Autodesk Inventor part; units mm, degrees
ref_plane "YZ Plane" through (0, 0, 0) normal (1, 0, 0) x (0, 1, 0)
ref_plane "XZ Plane" through (0, 0, 0) normal (0, 1, 0) x (-1, 0, 0)
ref_plane "XY Plane" through (0, 0, 0) normal (0, 0, 1) x (1, 0, 0)
sketch "Sketch1" plane through (0, 0, 0) normal (0, 0, 1) x (1, 0, 0)
  line L0 (49.9773, 11) -> (55.5082, 11)
  line L1 (-0.0227, 11) -> (-0.0227, 17)
  line L2 (-0.0227, 11) -> (-0.0227, 17)
  line L3 (-0.0227, 11) -> (-0.0227, 17)
  line L4 (-0.0227, 17) -> (55.5082, 17)
  line L5 (55.5082, 17) -> (55.5082, -83)
  line L6 (55.5082, -83) -> (-0.0227, -83)
  line L7 (-0.0227, -83) -> (-0.0227, 17)
  line L8 (55.5082, 17) -> (55.5082, 11)
  line L9 (55.5082, 17) -> (55.5082, 11)
  dimension "d16" = 100
extrude "Extrusion1" add sketch "Sketch1" along normal blind 6
sketch "Sketch2" plane through (0, 0, 6) normal (0, 0, 1) x (1, 0, 0)
  line L0 (49.9773, 11) -> (55.5082, 11)
  line L1 (49.9773, 17) -> (49.9773, 11)
  line L2 (29.9773, 17) -> (29.9773, 11)
  line L3 (29.9773, 11) -> (39.9773, 11)
  line L4 (39.9773, 11) -> (39.9773, 17)
  line L5 (49.9773, 11) -> (49.8773, 11)
  line L6 (49.8773, 11) -> (49.8773, 17)
  line L7 (49.8773, 17) -> (49.9773, 17)
  line L8 (49.9773, 17) -> (49.9773, 11)
  line L9 (39.9773, 11) -> (40.0773, 11)
  line L10 (40.0773, 11) -> (40.0773, 17)
  line L11 (40.0773, 17) -> (39.9773, 17)
  line L12 (39.9773, 17) -> (39.9773, 11)
  line L13 (29.9773, 11) -> (29.8773, 11)
  line L14 (29.8773, 11) -> (29.8773, 17)
  line L15 (29.8773, 17) -> (29.9773, 17)
  line L16 (29.9773, 17) -> (29.9773, 11)
  line L17 (9.9773, 17) -> (9.9773, 11)
  line L18 (19.9773, 11) -> (19.9773, 17)
  line L19 (9.9773, 11) -> (19.9773, 11)
  line L20 (19.9773, 11) -> (20.0773, 11)
  line L21 (20.0773, 11) -> (20.0773, 17)
  line L22 (20.0773, 17) -> (19.9773, 17)
  line L23 (19.9773, 17) -> (19.9773, 11)
  line L24 (9.9773, 11) -> (9.8773, 11)
  line L25 (9.8773, 11) -> (9.8773, 17)
  line L26 (9.8773, 17) -> (9.9773, 17)
  line L27 (9.9773, 17) -> (9.9773, 11)
  line L28 (55.5082, -83) -> (55.5082, 17)
  line L29 (39.9773, 11) -> (29.9773, 11)
  line L30 (19.9773, 11) -> (9.9773, 11)
  line L31 (49.9773, 11) -> (55.5082, 11)
  line L32 (-0.0227, 17) -> (-0.0227, -83)
  line L33 (55.5082, 17) -> (-0.0227, 17)
  point P0 (49.9, 0.06)
  point P1 (30.1, 0)
  point P2 (39.9, 0)
  point P3 (39.9, 0.03)
  point P4 (30.1, 2.97)
  point P5 (40, 0)
  point P6 (40, 0)
  point P7 (9.9773, 17)
  point P8 (19.9773, 17)
  point P9 (9.9773, 17)
  point P10 (39.9773, 17)
  point P11 (29.9773, 17)
  point P12 (49.9773, 17)
  dimension "d3" = 0.1
  dimension "d4" = 6
  dimension "d5" = 0.1
  dimension "d6" = 6
  dimension "d7" = 0.1
  dimension "d8" = 6
  dimension "d17" = 0.1
  dimension "d18" = 6
  dimension "d19" = 0.1
  dimension "d20" = 6
extrude "Extrusion2" cut sketch "Sketch2" against normal through all contours L5 L6 L7 L1 | L21 L20 L18 L22 | L4 L3 L2 L33 | L2 L13 L14 L15 | L18 L19 L17 L33 | L17 L24 L25 L26
ref_plane "Work Plane1" through (-0.0227, -33, 0) normal (0, -1, 0) x (1, 0, 0)
mirror "Mirror1" about plane through (-0.0227, -33, 0) normal (0, -1, 0) of "Extrusion2"
sketch "Sketch3" plane through (0, 0, 6) normal (0, 0, 1) x (1, 0, 0)
  line L0 (37.75, -5.4) -> (32.25, -5.4)
  line L1 (32.25, -5.4) -> (32.25, -3)
  line L2 (32.25, -3) -> (37.75, -3)
  line L3 (37.75, -3) -> (37.75, -5.4)
  line L4 (40.1, 7.6673) -> (40.1, 6)
  line L5 (40.1, 0) -> (29.9, 0)
  point P0 (0, 0)
  dimension "d21" = 5.5
  dimension "d22" = 2.4
  dimension "d23" = 2.35
  dimension "d24" = 3
extrude "Extrusion3" cut sketch "Sketch3" against normal through all
pattern_linear "Rectangular Pattern1" count 2 spacing 20 along (-1, 0, 0) of "Extrusion3"
mirror "Mirror2" about plane through (-0.0227, -33, 0) normal (0, -1, 0) of "Extrusion3", "Rectangular Pattern1"
properties part number "00_Baseplate_Simmo_side6_v2"
CAD build for the part. Positions are in the model's coordinates, mm. A direction names the side the tool comes from. Give positions to 0.01 mm unless a question says otherwise; leave off trailing zeros. Loops run counter-clockwise (first coordinate to the right, second up) from the corner with the lowest first, then second, coordinate; pieces in that order, holes last. Notation, with made-up numbers: M -4.75,22.5 L 15.25,22.5 A18 cw 15.25,36.5 Z; hole C 26.25,33 d10. An arc over 180 degrees is marked long. Answer in a Markdown table with one row per item. Add a question column.
Item 1: Probe probe 1 along Y at (x, z) = (36.5, 0.8); probe 2 along X at (y, z) = (-61.5, 0.45); probe 3 along Y at (x, z) = (11, 3). List the from-to ranges inside material, lowest first.
Item 2: Tool access for faces 4 (the face through (25, 17, 3)), 5 (the face through (35, -77, 3)), 6 (the face through (29.877, 14, 3)), 7 (the face through (35, -60.6, 3)), 8 (the face through (27, -32, 6)): list every direction of +Z, -Z, +X, -X, +Y, -Y with a clear straight run to the whole face (end or side of a thin tool).
Item 3: Mould opens along X. For faces 1 (the face through (5, -83, 3)), 2 (the face through (15, -3, 3)), 3 (the face through (55.508, -32, 3)) say: +X half, -X half, draft (parallel to the pull), parting line (faces both ways), or undercut.
Item 4: Drop flat-ended pins along their axis: P1, Ø3, axis at x = 18.5, z = 3.5, coming from the +Y side; P2, Ø1.6, axis at x = 14.5, z = 1.5, coming from the -Y side; P3, Ø12, axis at x = 41.5, y = -47.5, coming from the -Z side. Give the stop position or say it passes through.
Item 5: Band-saw the part on B-B on z = 3.15. Give the number of separate pieces and of enclosed holes in the cut face, then the cut area to 3 significant figures.
Item 6: Band-saw the part on A-A on x = 33.5. Give the cut face in (y, z), then the cut area to 3 significant figures.
Reply:
| question | item | result |
|---|---|---|
| 1 | probe 1 | y = -77 to -63, -60.6 to -5.4, -3 to 11 |
| 1 | probe 2 | x = -0.02 to 12.25, 17.75 to 32.25, 37.75 to 55.51 |
| 1 | probe 3 | y = -77 to 11 |
| 2 | face 4 | +Z, -Z, +X, -X, +Y |
| 2 | face 5 | +Z, -Z, -Y |
| 2 | face 6 | +Z, -Z, +Y |
| 2 | face 7 | +Z, -Z |
| 2 | face 8 | +Z, +X, -X, +Y, -Y |
| 3 | face 1 | draft |
| 3 | face 2 | undercut |
| 3 | face 3 | +X half |
| 4 | P1 | stops at y = 11 |
| 4 | P2 | stops at y = -77 |
| 4 | P3 | stops at z = 0 |
| 5 | separate pieces | 1 |
| 5 | enclosed holes | 4 |
| 5 | area | 5,260 mm^2 |
| 6 | outline | M -77,0 L -63,0 L -63,6 L -77,6 Z; M -60.6,0 L -5.4,0 L -5.4,6 L -60.6,6 Z; M -3,0 L 11,0 L 11,6 L -3,6 Z |
| 6 | area | 499 mm^2 |
